from build123d import *

# Parameters (mm, degrees)
F0_W     = 90
F0_H     = 9
F0_H_2   = 90
F0_R     = 2.5
F1_DEPTH = 10
F3_DEPTH = 5
F4_R     = 3.5
F4_R_2   = 2.5
F5_DEPTH = 25
F6_R     = 4
F6_R_2   = 2.1
F7_DEPTH = 4.5
F8_DEPTH = 25


with BuildPart() as f1:
    # F0 (on Top) → F1 (new body)
    with BuildSketch(Plane.XY):
        with Locations((0, -49.5)):
            Rectangle(F0_W, F0_H)
        Rectangle(F0_W, F0_H_2)
        with Locations((-37.5, -37.5)):
            Circle(F0_R, mode=Mode.SUBTRACT)
        with Locations((37.5, -37.5)):
            Circle(F0_R, mode=Mode.SUBTRACT)
        with Locations((-37.5, 37.5)):
            Circle(F0_R, mode=Mode.SUBTRACT)
        with Locations((37.5, 37.5)):
            Circle(F0_R, mode=Mode.SUBTRACT)
    extrude(amount=F1_DEPTH)

    # F2 (on face) → F3 (cut)
    with BuildSketch(Plane.XY.offset(10)):
        with BuildLine():
            Line((-33.9414238613, 30.1534489324), (-33.9414238613, 36.9554489324))
            ThreePointArc((-33.9414238613, 36.9554489324), (-37.5000142062, 41.1), (-41.0585718408, 36.9554208469))
            Line((-41.0585718408, 36.9554208469), (-41.0585718408, 30.153477018))
            ThreePointArc((-41.0585718408, 30.153477018), (-37.5000142062, 26.0088978648), (-33.9414238613, 30.1534489324))
        make_face()
        with BuildLine():
            Line((41.0578852383, 29.6284612117), (41.0578852383, 37.3796984459))
            ThreePointArc((41.0578852383, 37.3796984459), (37.2203682179, 41.0417420458), (33.8999927044, 36.9050517432))
            Line((33.8999927044, 36.9050517432), (33.8999927044, 30.1031079143))
            ThreePointArc((33.8999927044, 30.1031079143), (37.1506339605, 25.9717225558), (41.0578852383, 29.4885963107))
            Line((41.0578852383, 29.4885963107), (41.0578852383, 29.6284612117))
        make_face()
        with BuildLine():
            ThreePointArc((41.0578852383, 29.4885963107), (41.0585645452, 29.5585287612), (41.0578852383, 29.6284612117))
            Line((41.0578852383, 29.6284612117), (41.0578852383, 29.4885963107))
        make_face()
        with BuildLine():
            Line((-33.9414238613, -44.8465510676), (-33.9414238613, -38.0445510676))
            ThreePointArc((-33.9414238613, -38.0445510676), (-37.5000142062, -33.9), (-41.0585718408, -38.0445791531))
            Line((-41.0585718408, -38.0445791531), (-41.0585718408, -44.846522982))
            ThreePointArc((-41.0585718408, -44.846522982), (-37.5000142062, -48.9911021352), (-33.9414238613, -44.8465510676))
        make_face()
        with BuildLine():
            Line((41.0585761387, -44.8465510676), (41.0585761387, -38.0445510676))
            ThreePointArc((41.0585761387, -38.0445510676), (37.4999857938, -33.9), (33.9414281592, -38.0445791531))
            Line((33.9414281592, -38.0445791531), (33.9414281592, -44.846522982))
            ThreePointArc((33.9414281592, -44.846522982), (37.4999857938, -48.9911021352), (41.0585761387, -44.8465510676))
        make_face()
    extrude(amount=-F3_DEPTH, mode=Mode.SUBTRACT)

    # F4 (on face) → F5 (cut)
    with BuildSketch(Plane(origin=(0, 0, 0), x_dir=(1, 0, 0), z_dir=(0, 0, -1))):
        with Locations((-37.5, -37.5)):
            Circle(F4_R)
        with Locations((-37.5, -37.5)):
            Circle(F4_R_2, mode=Mode.SUBTRACT)
        with Locations((-37.5, 37.5)):
            Circle(F4_R)
        with Locations((-37.5, 37.5)):
            Circle(F4_R_2, mode=Mode.SUBTRACT)
        with Locations((37.5, 37.5)):
            Circle(F4_R)
        with Locations((37.5, 37.5)):
            Circle(F4_R_2, mode=Mode.SUBTRACT)
        with Locations((37.5, -37.5)):
            Circle(F4_R)
        with Locations((37.5, -37.5)):
            Circle(F4_R_2, mode=Mode.SUBTRACT)
    extrude(amount=-F5_DEPTH, mode=Mode.SUBTRACT)

    # F6 (on face) → F7 (cut)
    with BuildSketch(Plane(origin=(0, 0, 0), x_dir=(1, 0, 0), z_dir=(0, 0, -1))):
        with Locations((-29.51923199, -28.6538470536)):
            Circle(F6_R)
        with Locations((-29.51923199, -28.6538470536)):
            Circle(F6_R_2, mode=Mode.SUBTRACT)
        with Locations((28.6538470536, -29.51923199)):
            Circle(F6_R)
        with Locations((28.6538470536, -29.51923199)):
            Circle(F6_R_2, mode=Mode.SUBTRACT)
        with Locations((-28.6538470536, 29.51923199)):
            Circle(F6_R)
        with Locations((-28.6538470536, 29.51923199)):
            Circle(F6_R_2, mode=Mode.SUBTRACT)
        with Locations((29.51923199, 28.6538470536)):
            Circle(F6_R)
        with Locations((29.51923199, 28.6538470536)):
            Circle(F6_R_2, mode=Mode.SUBTRACT)
    extrude(amount=-F7_DEPTH, mode=Mode.SUBTRACT)

    # F8 (cut): faces of the model
    f8_faces = [f1.faces().sort_by_distance(p)[0] for p in [
        (-28.6538470536, -29.51923199, 0),
        (29.51923199, -28.6538470536, 0),
        (28.6538470536, 29.51923199, 0),
        (-29.51923199, 28.6538470536, 0),
    ]]
    extrude(f8_faces, amount=-F8_DEPTH, mode=Mode.SUBTRACT)


solid = f1.part
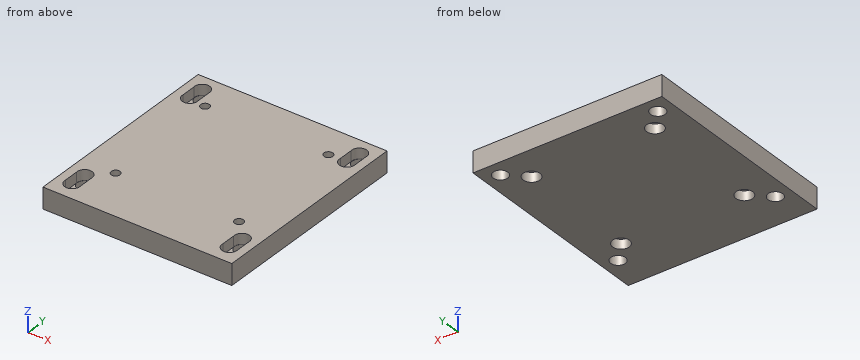
Read the model definition and answer for the solid it produces. Units are mm, in the model's axes. Coordinates: 2 decimals unless noted, no trailing zeros. Loops run counter-clockwise (first coordinate to the right, second up) from the corner with the lowest first, then second, coordinate; pieces in that order, holes last.
Q1. The part is cut by section B-B on z = 8.5. Give the number of separate pieces and of enclosed holes in the cut face, and give its area (3 significant figures).
Q2. Consider probe 1 along Y at (x, z) = (-37.5, 7); probe 2 along X at (y, z) = (34, 9.75); probe 3 along Y at (x, z) = (28, 5.25). Determine where each line is inside the solid, lowest interval first.
Q3. The part is cut by section C-C on x = 37.5. Write down the section's boundary in (y, z).
Q4. The part is cut by section A-A on x = -37.5. Write down the section's boundary in (y, z).
Q5. This flat-tipped pin is pushed along its axis until it touches: pin 1 Ø6.5 at (x, y) = (29.52, -28.65) entering from -Z. Where does it stop, or does it pass through?
Results below:
1. separate pieces: 1
1. enclosed holes: 8
1. area: 8,470 mm2
2. probe 1: y = -54 to -48.99, -33.9 to 26.01, 41.1 to 45
2. probe 2: x = -45 to -41.06, -33.94 to 33.9, 41.06 to 45
2. probe 3: y = -54 to -30.1, -27.2 to 27.52, 31.51 to 45
3. outline: (-54, 0) - (-41, 0) - (-41, 5) - (-48.99, 5) - (-48.99, 10) - (-54, 10) - close; (-34, 0) - (34, 0) - (34, 5) - (25.96, 5) - (25.96, 10) - (-33.9, 10) - (-33.9, 5) - (-34, 5) - close; (41, 0) - (45, 0) - (45, 10) - (41.05, 10) - (41.05, 5) - (41, 5) - close
4. outline: (-54, 0) - (-41, 0) - (-41, 5) - (-48.99, 5) - (-48.99, 10) - (-54, 10) - close; (-34, 0) - (34, 0) - (34, 5) - (26.01, 5) - (26.01, 10) - (-33.9, 10) - (-33.9, 5) - (-34, 5) - close; (41, 0) - (45, 0) - (45, 10) - (41.1, 10) - (41.1, 5) - (41, 5) - close
5. pin 1: stops at z = 4.5
